```python
from build123d import *

# Parameters (mm, degrees)
SKETCH_1_W      = 42
SKETCH_1_H      = 80
SKETCH_1_R      = 11
SKETCH_1_R_2    = 1.45
EXTRUDE_1_DEPTH = 4
CHAMFER_1_SIZE  = 5


with BuildPart() as part:
    # 草图1 → 凸台-拉伸1 (new body)
    with BuildSketch(Plane(origin=(0, 0, 0), x_dir=(1, 0, 0), z_dir=(0, 1, 0))):
        with Locations((21, 40)):
            Rectangle(SKETCH_1_W, SKETCH_1_H)
        with Locations(Location((21, 21, 0), (0, 0, 270))):
            Circle(SKETCH_1_R, mode=Mode.SUBTRACT)
        with Locations(Location((5.5, 36.5, 0), (0, 0, 270))):
            Circle(SKETCH_1_R_2, mode=Mode.SUBTRACT)
        with Locations(Location((5.5, 5.5, 0), (0, 0, 270))):
            Circle(SKETCH_1_R_2, mode=Mode.SUBTRACT)
        with Locations(Location((36.5, 36.5, 0), (0, 0, 270))):
            Circle(SKETCH_1_R_2, mode=Mode.SUBTRACT)
        with Locations(Location((36.5, 5.5, 0), (0, 0, 270))):
            Circle(SKETCH_1_R_2, mode=Mode.SUBTRACT)
        with BuildLine():
            Line((8, 74), (8, 61))
            ThreePointArc((8, 61), (6, 59), (4, 61))
            Line((4, 61), (4, 74))
            ThreePointArc((4, 74), (6, 76), (8, 74))
        make_face(mode=Mode.SUBTRACT)
        with BuildLine():
            Line((38, 74), (38, 61))
            ThreePointArc((38, 61), (36, 59), (34, 61))
            Line((34, 61), (34, 74))
            ThreePointArc((34, 74), (36, 76), (38, 74))
        make_face(mode=Mode.SUBTRACT)
    extrude(amount=EXTRUDE_1_DEPTH)

    # 倒角1
    chamfer_1_edges = [part.edges().sort_by_distance(p)[0] for p in [
        (0, 2, -80),
        (42, 2, -80),
        (42, 2, 0),
        (0, 2, 0),
    ]]
    chamfer(chamfer_1_edges, length=CHAMFER_1_SIZE)


solid = part.part
```
Part model, mm, in its own coordinate system. A direction names the side the tool comes from. Round coordinates to 2 decimals unless told otherwise and drop trailing zeros. Loops run counter-clockwise (first coordinate to the right, second up) from the corner with the lowest first, then second, coordinate; pieces in that order, holes last.
1. 3-axis set-ups, long thin cutter, end or side, ignore diameter. For faces 1 (the face through (3, 2, -2)), 2 (the face through (38, 2, -68)): which of +Z, -Z, +X, -X, +Y, -Y reach the whole face in a straight line?
Solutions:
face 1: +Z, -X, +Y, -Y
face 2: +Y, -Y
2. Slice it at D-D (y = 3.05). Give the cut face in (x, z), and give its area (3 significant figures).
Solutions:
outline: (0, -75) - (5, -80) - (37, -80) - (42, -75) - (42, -5) - (37, 0) - (5, 0) - (0, -5) - close; hole (4, -74) arc R2 ccw to (8, -74) - (8, -61) arc R2 ccw to (4, -61) - close; hole circle Ø2.9 at (5.5, -36.5); hole circle Ø2.9 at (5.5, -5.5); hole circle Ø22 at (21, -21); hole (34, -74) arc R2 ccw to (38, -74) - (38, -61) arc R2 ccw to (34, -61) - close; hole circle Ø2.9 at (36.5, -36.5); hole circle Ø2.9 at (36.5, -5.5)
area: 2,770 mm2
3. Drill centre lines: line 1 along X through (y, z) = (0.85, -5.5); line 2 along X through (y, z) = (1, -21); line 3 along X through (y, z) = (1.55, -6.5). Where is each one in solid material? Low to high.
Solutions:
line 1: x = 0 to 4.05, 6.95 to 35.05, 37.95 to 42
line 2: x = 0 to 10, 32 to 42
line 3: x = 0 to 4.45, 6.55 to 35.45, 37.55 to 42
4. Two-plate mould, pull along X, no slides. Class faces 3 (the face through (21, 4, -41)), 4 (the face through (3, 2, -78)), 5 (the face through (6, 2, -76)): pulls with the +X half, pulls with the -X half, needs draft (parallel to the pull), parting line crosses it, or undercut.
Solutions:
face 3: needs draft
face 4: pulls with the -X half
face 5: undercut
5. Slice it at A-A (z = -21). Give the cut face in (x, y), and give its area (3 significant figures).
Solutions:
outline: (0, 0) - (10, 0) - (10, 4) - (0, 4) - close; (32, 0) - (42, 0) - (42, 4) - (32, 4) - close
area: 80.0 mm2
6. Slice it at C-C (x = 21). Give the cut face in (y, z), and give its area (3 significant figures).
Solutions:
outline: (0, -80) - (4, -80) - (4, -32) - (0, -32) - close; (0, -10) - (4, -10) - (4, 0) - (0, 0) - close
area: 232 mm2
7. Slice it at B-B (z = -36.5). Give the cut face in (x, y), and give its area (3 significant figures).
Solutions:
outline: (0, 0) - (4.05, 0) - (4.05, 4) - (0, 4) - close; (6.95, 0) - (35.05, 0) - (35.05, 4) - (6.95, 4) - close; (37.95, 0) - (42, 0) - (42, 4) - (37.95, 4) - close
area: 145 mm2
8. Flat gauge pin, fed straight in: pin 1 (1.7 mm diameter, centred on x = 5.5, z = -36.5, fed in from +Y). Where does the tip first touch, or does it go through?
Solutions:
pin 1: passes through
